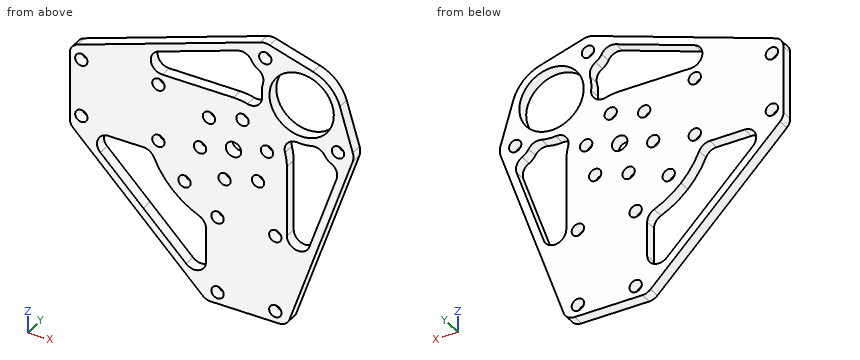
from build123d import *

# Parameters (mm, degrees)
BOSS_EXTRUDE1_DEPTH      = 3
M3_CLEARANCE_HOLE1_D     = 3.2
M3_CLEARANCE_HOLE2_D     = 3.2
F_4_0_4_DIAMETER_HOLE1_D = 4
CUT_EXTRUDE3_DEPTH       = 3
FILLET5_R                = 3
M3_CLEARANCE_HOLE3_D     = 3.2
CUT_EXTRUDE4_START       = -3
CUT_EXTRUDE4_DEPTH       = 3
BOSS_EXTRUDE2_START      = -3
SKETCH17_R               = 8.35
BOSS_EXTRUDE2_DEPTH      = 3
BOSS_EXTRUDE3_START      = -3
BOSS_EXTRUDE3_DEPTH      = 3
M3_CLEARANCE_HOLE4_D     = 3.2
CUT_EXTRUDE5_START       = -3
CUT_EXTRUDE5_DEPTH       = 3
FILLET6_R                = 3
FILLET7_R                = 3


# Some blends are built 0.0001 mm under size
with BuildPart() as part:
    # Sketch2 → Boss-Extrude1 (new body)
    with BuildSketch(Plane(origin=(0, 0, 0), x_dir=(1, 0, 0), z_dir=(0, 1, 0))):
        with BuildLine():
            Line((-16.5, -13.85), (-42.5, -13.85))
            Line((-42.5, -13.85), (-42.5, 7.15))
            Line((-42.5, 7.15), (-24.825, 24.825))
            Line((-24.825, 24.825), (25.724873734, -25.724873734))
            Line((25.724873734, -25.724873734), (16.974873734, -34.474873734))
            ThreePointArc((16.974873734, -34.474873734), (14.482141695, -35.49995444), (12, -34.449489743))
            Line((12, -34.449489743), (12, -39))
            Line((12, -39), (-12, -39))
            Line((-12, -39), (-12, -34.449489743))
            ThreePointArc((-12, -34.449489743), (-17.17260394, -34.259908888), (-16.5, -29.127718677))
            Line((-16.5, -29.127718677), (-16.5, -13.85))
        make_face()
    extrude(amount=BOSS_EXTRUDE1_DEPTH)

    # Mirror5: part across plane


with BuildPart() as part_1:
    add(part.part)
    add(part.part.mirror(Plane(origin=(25.724873734, 3, 25.724873734), x_dir=(0.7071067811865465, 0, 0.7071067811865487), z_dir=(-0.7071067811865486, 0, 0.7071067811865465))))

    # M3 Clearance Hole1 (through all)
    with Locations(Plane(origin=(0, 3, 0), x_dir=(1, 0, 0), z_dir=(0, 1, 0))):
        with Locations((-39.5, 4.15), (-19.5, 4.15), (-19.5, -10.85), (-39.5, -10.85), (-4.15, 19.5), (-4.15, 39.5), (10.85, 39.5), (10.85, 19.5)):
            Hole(M3_CLEARANCE_HOLE1_D / 2)

    # M3 Clearance Hole2 (through all)
    with Locations(Plane(origin=(0, 3, 0), x_dir=(1, 0, 0), z_dir=(0, 1, 0))):
        with Locations((-2.329371406, 8.693332437), (6.363961031, 6.363961031), (8.693332437, -2.329371406), (2.329371406, -8.693332437), (-6.363961031, -6.363961031), (-8.693332437, 2.329371406)):
            Hole(M3_CLEARANCE_HOLE2_D / 2)

    # Ø4.0 (4) Diameter Hole1 (through all)
    with Locations(Plane(origin=(0, 3, 0), x_dir=(1, 0, 0), z_dir=(0, 1, 0))):
        with Locations((0, 0)):
            Hole(F_4_0_4_DIAMETER_HOLE1_D / 2)

    # Sketch13 → Cut-Extrude3 (cut)
    with BuildSketch(Plane(origin=(0, 3, 0), x_dir=(1, 0, 0), z_dir=(0, 1, 0))):
        with BuildLine():
            Line((-39.671572875, 7.15), (-21.333717444, 7.15))
            ThreePointArc((-21.333717444, 7.15), (-19.129970762, 11.844586048), (-15.909902577, 15.909902577))
            Line((-15.909902577, 15.909902577), (-23.410786438, 23.410786438))
            Line((-23.410786438, 23.410786438), (-39.671572875, 7.15))
        make_face()
    cut_extrude3 = extrude(amount=-CUT_EXTRUDE3_DEPTH, mode=Mode.SUBTRACT)

    # Mirror6: Cut-Extrude3 across plane
    add(cut_extrude3.mirror(Plane(origin=(0, -28.792883686, 0), x_dir=(0.7071067811865467, 0, 0.7071067811865482), z_dir=(-0.7071067811865482, 0, 0.7071067811865468))), mode=Mode.SUBTRACT)

    # Fillet5
    fillet5_edges = [part_1.edges().sort_by_distance(p)[0] for p in [
        (-21.333717444, 1.5, -7.15),
        (-39.671572875, 1.5, -7.15),
        (-7.15, 1.5, -21.333717444),
        (-7.15, 1.5, -39.671572875),
    ]]
    fillet(fillet5_edges, radius=FILLET5_R)

    # M3 Clearance Hole3 (through all)
    with Locations(Plane(origin=(0, 3, 0), x_dir=(1, 0, 0), z_dir=(0, 1, 0))):
        with Locations((-12.727922061, 12.727922061)):
            Hole(M3_CLEARANCE_HOLE3_D / 2)

    # Sketch16 → Cut-Extrude4 (cut)
    with BuildSketch(Plane(origin=(0, 3, 0), x_dir=(1, 0, 0), z_dir=(0, 1, 0)).offset(CUT_EXTRUDE4_START)):
        with BuildLine():
            Line((-16.5, -13.85), (-10.493288043, -8.808002387))
            ThreePointArc((-10.493288043, -8.808002387), (9.687362902, -9.687362902), (8.808002387, 10.493288043))
            Line((8.808002387, 10.493288043), (13.85, 16.5))
            Line((13.85, 16.5), (29.127718677, 16.5))
            ThreePointArc((29.127718677, 16.5), (34.259908888, 17.17260394), (34.449489743, 12))
            Line((34.449489743, 12), (39, 12))
            Line((39, 12), (39, -12))
            Line((39, -12), (34.449489743, -12))
            ThreePointArc((34.449489743, -12), (35.49995444, -14.482141695), (34.474873734, -16.974873734))
            Line((34.474873734, -16.974873734), (16.974873734, -34.474873734))
            ThreePointArc((16.974873734, -34.474873734), (14.482141695, -35.49995444), (12, -34.449489743))
            Line((12, -34.449489743), (12, -39))
            Line((12, -39), (-12, -39))
            Line((-12, -39), (-12, -34.449489743))
            ThreePointArc((-12, -34.449489743), (-17.17260394, -34.259908888), (-16.5, -29.127718677))
            Line((-16.5, -29.127718677), (-16.5, -13.85))
        make_face()
    extrude(amount=CUT_EXTRUDE4_DEPTH, mode=Mode.SUBTRACT)

    # Sketch17 → Boss-Extrude2 (add)
    with BuildSketch(Plane(origin=(0, 3, 0), x_dir=(1, 0, 0), z_dir=(0, 1, 0)).offset(BOSS_EXTRUDE2_START)):
        with BuildLine():
            Line((-16.5, -13.85), (13.483684727, -27.139856987))
            ThreePointArc((13.483684727, -27.139856987), (24.996224715, -24.996224715), (27.139856987, -13.483684727))
            Line((27.139856987, -13.483684727), (13.85, 16.5))
            Line((13.85, 16.5), (8.808002387, 10.493288043))
            ThreePointArc((8.808002387, 10.493288043), (9.687362902, -9.687362902), (-10.493288043, -8.808002387))
            Line((-10.493288043, -8.808002387), (-16.5, -13.85))
        make_face()
        with Locations(Location((17.67766953, -17.67766953, 0), (0, 0, 270))):
            Circle(SKETCH17_R, mode=Mode.SUBTRACT)
    extrude(amount=BOSS_EXTRUDE2_DEPTH)

    # Sketch18 → Boss-Extrude3 (add)
    with BuildSketch(Plane(origin=(0, 3, 0), x_dir=(1, 0, 0), z_dir=(0, 1, 0)).offset(BOSS_EXTRUDE3_START)):
        with BuildLine():
            Line((30.898968891, -6.933633811), (13.85, 42.5))
            Line((13.85, 42.5), (13.85, 16.5))
            Line((13.85, 16.5), (27.139856987, -13.483684727))
            ThreePointArc((27.139856987, -13.483684727), (28.006636609, -17.018170416), (27.596413119, -20.634192082))
            Line((27.596413119, -20.634192082), (30.950875914, -9.380411412))
            ThreePointArc((30.950875914, -9.380411412), (31.116645257, -8.152955318), (30.898968891, -6.933633811))
        make_face()
        with BuildLine():
            Line((-42.5, -13.85), (-16.5, -13.85))
            Line((-16.5, -13.85), (13.483684727, -27.139856987))
            ThreePointArc((13.483684727, -27.139856987), (17.018170416, -28.006636609), (20.634192082, -27.596413119))
            Line((20.634192082, -27.596413119), (9.380411412, -30.950875914))
            ThreePointArc((9.380411412, -30.950875914), (8.152955318, -31.116645257), (6.933633811, -30.898968891))
            Line((6.933633811, -30.898968891), (-42.5, -13.85))
        make_face()
    extrude(amount=BOSS_EXTRUDE3_DEPTH)

    # M3 Clearance Hole4 (through all)
    with Locations(Plane(origin=(0, 3, 0), x_dir=(1, 0, 0), z_dir=(0, 1, 0))):
        with Locations((8.237794001, -27.117545059), (27.117545059, -8.237794001)):
            Hole(M3_CLEARANCE_HOLE4_D / 2)

    # Sketch21 → Cut-Extrude5 (cut)
    with BuildSketch(Plane(origin=(0, 3, 0), x_dir=(1, 0, 0), z_dir=(0, 1, 0)).offset(CUT_EXTRUDE5_START)):
        with BuildLine():
            Line((13.85, 36.365784234), (27.878821119, -4.310904805))
            ThreePointArc((27.878821119, -4.310904805), (25.451546124, -4.601250649), (23.646518046, -6.249837391))
            ThreePointArc((23.646518046, -6.249837391), (22.205721923, -7.524489916), (20.286938067, -7.661970967))
            ThreePointArc((20.286938067, -7.661970967), (15.946603087, -7.473459175), (11.911266823, -9.082839698))
            Line((11.911266823, -9.082839698), (11.104995265, -8.27656814))
            ThreePointArc((11.104995265, -8.27656814), (13.145848858, -4.359949288), (13.85, 0))
            Line((13.85, 0), (13.85, 36.365784234))
        make_face()
        with BuildLine():
            Line((0, -13.85), (-36.365784234, -13.85))
            Line((-36.365784234, -13.85), (4.310904805, -27.878821119))
            ThreePointArc((4.310904805, -27.878821119), (4.601250649, -25.451546124), (6.249837391, -23.646518046))
            ThreePointArc((6.249837391, -23.646518046), (7.524489916, -22.205721923), (7.661970967, -20.286938067))
            ThreePointArc((7.661970967, -20.286938067), (7.473459175, -15.946603087), (9.082839698, -11.911266823))
            Line((9.082839698, -11.911266823), (8.27656814, -11.104995265))
            ThreePointArc((8.27656814, -11.104995265), (4.359949288, -13.145848858), (0, -13.85))
        make_face()
    extrude(amount=CUT_EXTRUDE5_DEPTH, mode=Mode.SUBTRACT)

    # Fillet6
    # the kernel refuses this fillet: 3 mm, written as the material it adds along each edge
    with BuildSketch(Plane(origin=(13.85, 0, -36.365784234), x_dir=(0, 0, 1), z_dir=(0, 1, 0)), Plane(origin=(-36.365784234, 0, 13.85), x_dir=(0.945355958029755, 0, 0.3260400475672341), z_dir=(0, 1, 0))) as fillet6_piece_1:
        with BuildLine():
            CenterArc((FILLET6_R * 5.96661659371, FILLET6_R), FILLET6_R, 109.02859786, 160.97140214)
            Line((FILLET6_R * 5.64057654615, FILLET6_R * 1.94535595803), (FILLET6_R * 5.63405574519, FILLET6_R * 1.96426307719))
            Line((FILLET6_R * 5.63405574519, FILLET6_R * 1.96426307719), (-FILLET6_R * 0.00652080095135, FILLET6_R * 0.0189071191606))
            Line((-FILLET6_R * 0.00652080095135, FILLET6_R * 0.0189071191606), (0, -FILLET6_R * 0.02))
            Line((0, -FILLET6_R * 0.02), (FILLET6_R * 5.96661659371, -FILLET6_R * 0.02))
            Line((FILLET6_R * 5.96661659371, -FILLET6_R * 0.02), (FILLET6_R * 5.96661659371, 0))
        make_face()
    extrude(amount=3)
    with BuildSketch(Plane(origin=(27.878821119, 0, 4.310904805), x_dir=(-0.32604004756723476, 0, -0.9453559580297546), z_dir=(0, 1, 0))) as fillet6_piece_2:
        with BuildLine():
            CenterArc((3.464101615, 3), FILLET6_R, 188.213210702, 81.786789298)
            Line((0.494871659, 2.571428571), (0.43548706, 2.562857143))
            ThreePointArc((0.43548706, 2.562857143), (0.404901579, 1.255409988), (-0.051961524, 0.03))
            Line((-0.051961524, 0.03), (0, -0.06))
            Line((0, -0.06), (3.464101615, -0.06))
            Line((3.464101615, -0.06), (3.464101615, 0))
        make_face()
    extrude(amount=3)
    with BuildSketch(Plane(origin=(11.104995265, 0, 8.27656814), x_dir=(0.7071067811869455, 0, 0.7071067811861494), z_dir=(0, 1, 0))) as fillet6_piece_3:
        with BuildLine():
            CenterArc((2.481144361, 2.683649746), FILLET6_R, 196.13857285, 47.312103401)
            Line((-0.400632365, 1.849765518), (-0.458267899, 1.833087834))
            ThreePointArc((-0.458267899, 1.833087834), (-0.227322426, 0.919033599), (-0.059371126, -0.00866426))
            Line((-0.059371126, -0.00866426), (0, -0.06))
            ThreePointArc((0, -0.06), (0.570120087, -0.06), (1.113422089, -0.053672995))
            Line((1.113422089, -0.053672995), (1.140240173, 0))
        make_face()
    extrude(amount=3)
    with BuildSketch(Plane(origin=(8.27656814, 0, 11.104995265), x_dir=(-0.8407620685724203, 0, 0.5414047876125816), z_dir=(0, 1, 0))) as fillet6_piece_4:
        with BuildLine():
            CenterArc((2.097634461, 2.992988969), FILLET6_R, 218.770003629, 47.312103401)
            Line((-0.241363262, 1.114401825), (-0.288143216, 1.076830083))
            ThreePointArc((-0.288143216, 1.076830083), (-0.179322004, 0.544500259), (-0.058640373, -0.012700654))
            Line((-0.058640373, -0.012700654), (0.004099611, -0.059859779))
            ThreePointArc((0.004099611, -0.059859779), (0.946326947, -0.027632406), (1.888554283, -0.059859779))
            Line((1.888554283, -0.059859779), (1.892653895, 0))
        make_face()
    extrude(amount=3)
    with BuildSketch(Plane(origin=(4.310904805, 0, 27.878821119), x_dir=(0.14150948766511262, 0, -0.98993689945408), z_dir=(0, 1, 0))) as fillet6_piece_5:
        with BuildLine():
            CenterArc((3.600595189, 2.834733548), FILLET6_R, 169.106605351, 81.786789298)
            Line((0.654653671, 3.401680257), (0.59573484, 3.413019191))
            Line((0.59573484, 3.413019191), (-0.05891883, 0.011338934))
            Line((-0.05891883, 0.011338934), (0.01963961, -0.056694671))
            ThreePointArc((0.01963961, -0.056694671), (1.309307341, 0.16035527), (2.598975073, -0.056694671))
            Line((2.598975073, -0.056694671), (2.618614683, 0))
        make_face()
    extrude(amount=3)

    # Fillet7
    fillet7_edges = [part_1.edges().sort_by_distance(p)[0] for p in [
        (11.911266823, 1.5, 9.082839698),
        (9.082839698, 1.5, 11.911266823),
        (-42.5, 1.5, -7.15),
        (-7.15, 1.5, -42.5),
        (13.85, 1.5, -42.5),
        (-42.5, 1.5, 13.85),
    ]]
    fillet(fillet7_edges, radius=FILLET7_R - 0.0001)  # a hair under: the kernel refuses the full size


solid = part_1.part
Can you work these out from the model? Positions are in its coordinate system, mm. Round coordinates to 2 decimals unless told otherwise and drop trailing zeros. Order: outer loops, then holes, each group sorted by start corner. A loop starts at its lowest first (then second) coordinate and runs counter-clockwise, first axis right, second up. Notation, with made-up numbers: (17, 34.5) -> (61, 34.5) arc R24 ccw to (61, 61.5) -> close; hole circle Ø8 at (-33.75, 13.5). An arc over 180 degrees is marked (long way). Write each question's results on one line, items separated by ' | '. Start each with the question number.
Item 1: Will these pins go through, and if not, where does the flat tip stop? pin 1 (0.9 mm diameter, centred on y = 2, z = -8, fed in from +X); pin 2 (1 mm diameter, centred on y = 2, z = -16, fed in from -X).
Item 2: Please list where these lines run through material, in increasing order: L1, parallel to Z at x = -10, y = 2.05; L2, parallel to X at y = 2.9, z = -17.5; L3, parallel to Z at x = -1.5, y = 1.55.
Item 3: If we section it at A-A, the plane z = 22: Write out the boundary of the cut face in (x, y), then the cut area to 3 significant figures.
Item 4: If we section it at D-D, the plane y = 1.4: State how many separate pieces and enclosed holes the cut face has, then the cut area to 3 significant figures.
Item 5: If we section it at B-B, the plane z = -30: Write out the boundary of the cut face in (x, y).
Item 6: If we section it at C-C, the plane z = -39.5: Write out the boundary of the cut face in (x, y), then the cut area to 3 significant figures.
Results:
1) pin 1: stops at x = 25.9 | pin 2: stops at x = -34.15
2) L1: z = -39.65 to -35.43, -20.16 to -3.25, -1.41 to 13.85, 22.94 to 25.06 | L2: x = -32.15 to -29.32, -14.14 to 13.85, 20.36 to 22.47 | L3: z = -42.5 to -10.06, -7.33 to -1.32, 1.32 to 13.85, 25.87 to 27.99
3) outline: (-18.87, 0) -> (-12.73, 0) -> (-12.73, 3) -> (-18.87, 3) -> close; (7.6, 0) -> (10.53, 0) -> (10.53, 3) -> (7.6, 3) -> close; (24.82, 0) -> (27.08, 0) -> (27.08, 3) -> (24.82, 3) -> close | area: 34.0 mm2
4) separate pieces: 1 | enclosed holes: 22 | area: 2,520 mm2
5) outline: (-19.65, 0) -> (-16.82, 0) -> (-16.82, 3) -> (-19.65, 3) -> close; (-7.15, 0) -> (18.16, 0) -> (18.16, 3) -> (-7.15, 3) -> close
6) outline: (-10.15, 0) -> (-5.75, 0) -> (-5.75, 3) -> (-10.15, 3) -> close; (-2.55, 0) -> (9.25, 0) -> (9.25, 3) -> (-2.55, 3) -> close; (12.45, 0) -> (14.88, 0) -> (14.88, 3) -> (12.45, 3) -> close | area: 55.9 mm2
